from build123d import *

# Parameters (mm, degrees)
SKETCH_1_R      = 9
SKETCH_1_R_2    = 1.5
EXTRUDE_1_DEPTH = 10


with BuildPart() as part:
    # Эскиз1 → Бобышка-Вытянуть1 (new body)
    with BuildSketch(Plane(origin=(0, 0, 0), x_dir=(1, 0, 0), z_dir=(0, 1, 0))):
        with BuildLine():
            Line((-31.5, 0), (-31.5, -10))
            Line((-31.5, -10), (-14.361406616, -10))
            ThreePointArc((-14.361406616, -10), (0, -17.5), (14.361406616, -10))
            Line((14.361406616, -10), (31.5, -10))
            Line((31.5, -10), (31.5, 0))
            Line((31.5, 0), (41.5, 0))
            Line((41.5, 0), (41.5, 5))
            Line((41.5, 5), (16.770509831, 5))
            ThreePointArc((16.770509831, 5), (0, 17.5), (-16.770509831, 5))
            Line((-16.770509831, 5), (-41.5, 5))
            Line((-41.5, 5), (-41.5, 0))
            Line((-41.5, 0), (-31.5, 0))
        make_face()
        with Locations(Location((0, 0, 0), (0, 0, 270))):
            Circle(SKETCH_1_R, mode=Mode.SUBTRACT)
        with Locations(Location((-8.838834765, 8.838834765, 0), (0, 0, 270))):
            Circle(SKETCH_1_R_2, mode=Mode.SUBTRACT)
        with Locations(Location((8.838834765, 8.838834765, 0), (0, 0, 270))):
            Circle(SKETCH_1_R_2, mode=Mode.SUBTRACT)
        with Locations(Location((8.838834765, -8.838834765, 0), (0, 0, 270))):
            Circle(SKETCH_1_R_2, mode=Mode.SUBTRACT)
        with Locations(Location((-8.838834765, -8.838834765, 0), (0, 0, 270))):
            Circle(SKETCH_1_R_2, mode=Mode.SUBTRACT)
    extrude(amount=EXTRUDE_1_DEPTH)


solid = part.part
Input: part model. Units: mm. Frame: model coordinates. A direction names the side the tool comes from. Give positions to 0.01 mm unless a question says otherwise; leave off trailing zeros. Write each loop counter-clockwise with the first axis right and the second up, starting at its lowest first coordinate (ties: lowest second). Pieces come first, ordered by that corner, then holes.
Q1. Pull-direction query (Z, two-part tool) for faces 1 (the face through (-23, 5, 10)), 2 (the face through (-29, 5, -5)), 3 (the face through (-10.3, 4.9, 8.5)); classes: pulls with the +Z half, pulls with the -Z half, needs draft (parallel to the pull), parting line crosses it, or undercut.
Q2. Section C-C, the plane z = -3. Output: boundary loops of the cut face in (x, y), plus the area to 3 significant figures.
Q3. Section A-A, the plane x = 0. Output: boundary loops of the cut face in (y, z), plus the area to 3 significant figures.
Q4. First-contact query: P1, Ø5, axis at x = -38, y = 3.5, coming from the +Z side; P2, Ø4, axis at y = 6.5, z = -10, coming from the +X side; P3, Ø1.5, axis at y = 3.5, z = -13.5, coming from the +X side. Flat tips, straight axial feed; report the tip coordinate or a pass-through.
Q5. Section B-B, the plane y = 1. Output: boundary loops of the cut face in (x, z).
Q6. Set-up query: faces 4 (the face through (29, 5, -5)), 5 (the face through (-37, 5, 0)), 6 (the face through (23, 5, 10)), 7 (the face through (-10, 0, 0)). Return all of +Z, -Z, +X, -X, +Y, -Y with unobstructed straight access to the full face (end or side cutting, diameter ignored); none if empty.
Q7. Material intervals for probe 1 along X at (y, z) = (4, 7.5); probe 2 along Z at (x, y) = (-8, 6.5); probe 3 along Z at (x, y) = (-20.5, 2.5), sorted ascending.
Q8. Section D-D, the plane x = 19. Output: boundary loops of the cut face in (y, z), plus the area to 3 significant figures.
Filled in:
1. face 1: pulls with the +Z half
1. face 2: pulls with the -Z half
1. face 3: undercut
2. outline: (-41.5, 0) - (-8.49, 0) - (-8.49, 10) - (-41.5, 10) - close; (8.49, 0) - (41.5, 0) - (41.5, 10) - (8.49, 10) - close
2. area: 660 mm2
3. outline: (0, -17.5) - (10, -17.5) - (10, -9) - (0, -9) - close; (0, 9) - (10, 9) - (10, 17.5) - (0, 17.5) - close
3. area: 170 mm2
4. P1: stops at z = 0
4. P2: stops at x = 15.56
4. P3: stops at x = 11.99
5. outline: (-41.5, -5) - (-16.77, -5) arc R17.5 ccw to (16.77, -5) - (41.5, -5) - (41.5, 0) - (31.5, 0) - (31.5, 10) - (14.36, 10) arc R17.5 ccw to (-14.36, 10) - (-31.5, 10) - (-31.5, 0) - (-41.5, 0) - close; hole circle Ø3 at (-8.84, -8.84); hole circle Ø3 at (-8.84, 8.84); hole circle Ø18 at (0, 0); hole circle Ø3 at (8.84, -8.84); hole circle Ø3 at (8.84, 8.84)
6. face 4: -Z, +X, +Y, -Y
6. face 5: +Z, -X, +Y, -Y
6. face 6: +Z, +X, +Y, -Y
6. face 7: +Z, -Z, +X, -X, -Y
7. probe 1: x = -31.5 to -9.52, -8.16 to -4.97, 4.97 to 8.16, 9.52 to 31.5
7. probe 2: z = -15.56 to -10.08, -7.6 to -4.12, 4.12 to 7.6, 10.08 to 15.56
7. probe 3: z = -5 to 10
8. outline: (0, -5) - (10, -5) - (10, 10) - (0, 10) - close
8. area: 150 mm2
